Autodesk Inventor part; units mm, degrees
ref_plane "YZ Plane" through (0, 0, 0) normal (1, 0, 0) x (0, 1, 0)
ref_plane "XZ Plane" through (0, 0, 0) normal (0, 1, 0) x (-1, 0, 0)
ref_plane "XY Plane" through (0, 0, 0) normal (0, 0, 1) x (1, 0, 0)
sketch "스케치1" plane through (0, 0, 0) normal (0, 1, 0) x (-1, 0, 0)
  line L0 (-150, 125) -> (-150, -175)
  line L1 (-150, -175) -> (150, -175)
  line L2 (150, -175) -> (150, 125)
  line L3 (150, 125) -> (100, 125)
  line L4 (100, 125) -> (100, 175)
  line L5 (100, 175) -> (-100, 175)
  line L6 (-100, 175) -> (-100, 125)
  line L7 (-100, 125) -> (-150, 125)
  point P0 (0, 0)
  dimension "d3" = 300
  dimension "d4" = 150
  dimension "d8" = 350
  dimension "d10" = 175
  dimension "d11" = 50
extrude "돌출1" add sketch "스케치1" along normal blind 10
sketch "스케치3" plane through (0, 0, 0) normal (0, 0, 1) x (1, 0, 0)
  line L0 (150, 10) -> (-150, 10)
  line L1 (-125, 10) -> (-84.6452, 58.0929)
  line L2 (-59.1104, 70) -> (59.1104, 70)
  line L3 (100, 0) -> (100, 10)
  line L4 (84.6452, 58.0929) -> (125, 10)
  line L5 (0, 0) -> (0, 70)
  arc A0 (-59.1104, 70) -> (-84.6452, 58.0929) centre (-59.1104, 36.6667) ccw
  arc A1 (84.6452, 58.0929) -> (59.1104, 70) centre (59.1104, 36.6667) ccw
  line L6 (125, 10) -> (-125, 10)
  point P0 (-74.654, 70)
  point P1 (74.654, 70)
  point P2 (125, 10)
  dimension "d15" = 130
  dimension "d17" = 33.3333
  dimension "d18" = 33.3333
  dimension "d19" = 300
  dimension "d22" = 250
  dimension "d24" = 60
  dimension "d25" = 0
sketch "스케치4" plane through (0, 0, 0) normal (1, 0, 0) x (0, 1, 0)
  line L0 (70, -175) -> (70, 59.1104)
  line L1 (58.0929, 84.6452) -> (10, 125)
  line L2 (10, 175) -> (10, 125)
  line L3 (10, -175) -> (10, 125)
  line L4 (70, -175) -> (10, -175)
  arc A0 (70, 59.1104) -> (58.0929, 84.6452) centre (36.6667, 59.1104) ccw
  point P0 (0, 0)
  dimension "d27" = 130
  dimension "d28" = 33.3333
  dimension "d29" = 60
extrude "돌출3" add sketch "스케치3" against normal up to surface (175 mm away)
sketch "스케치5" plane through (0, 10, 0) normal (0, 1, 0) x (1, 0, 0)
  line L0 (125, 175) -> (125, 0)
  line L1 (125, 0) -> (-125, 0)
  line L2 (-125, 0) -> (-125, 175)
  line L3 (-125, 175) -> (-150, 175)
  line L4 (-150, 175) -> (-150, -125)
  line L5 (-150, -125) -> (-100, -125)
  line L6 (-100, -125) -> (-100, -175)
  line L7 (-100, -175) -> (100, -175)
  line L8 (100, -175) -> (100, -125)
  line L9 (100, -125) -> (150, -125)
  line L10 (150, -125) -> (150, 175)
  line L11 (150, 175) -> (125, 175)
  line L12 (66, -151) -> (-66, -151)
  line L13 (-76, -141) -> (-76, -111)
  line L14 (-86, -101) -> (-116, -101)
  line L15 (-126, -91) -> (-126, -24)
  line L16 (-126, -24) -> (126, -24)
  line L17 (126, -24) -> (126, -91)
  line L18 (116, -101) -> (86, -101)
  line L19 (76, -111) -> (76, -141)
  arc A0 (86, -101) -> (76, -111) centre (86, -111) ccw
  arc A1 (-76, -111) -> (-86, -101) centre (-86, -111) ccw
  arc A2 (116, -101) -> (126, -91) centre (116, -91) ccw
  arc A3 (-126, -91) -> (-116, -101) centre (-116, -91) ccw
  arc A4 (-76, -141) -> (-66, -151) centre (-66, -141) ccw
  arc A5 (66, -151) -> (76, -141) centre (66, -141) ccw
  point P0 (0, 0)
  dimension "d34" = 24
  dimension "d35" = 10
  dimension "d36" = 10
equation "\"d17\" = 0.5 * d14"
equation "\"d18\" = d17"
equation "\"d22\" = 0.833333 * d19"
equation "\"d24\" = 0.2 * d19"
equation "\"d27\" = d15"
equation "\"d28\" = d17"
equation "\"d29\" = d24"
equation "\"d36\" = d35"
equation "\"d14\" = 0.333333 * d16"
properties part number "cap2"
Design review of the part built by this model. Coordinates are the model's own, in mm. A direction names the side the tool comes from. Give positions to 0.01 mm unless a question says otherwise; leave off trailing zeros. Order: outer loops, then holes, each group sorted by start corner. A loop starts at its lowest first (then second) coordinate and runs counter-clockwise, first axis right, second up. Notation, with made-up numbers: (72, 24) -> (89, 24) arc R14 cw to (89, 48) -> close; hole circle Ø7 at (36, 14.25). An arc over 180 degrees is marked (long way). Write each question's results on one line, items separated by ' | '. Start each with the question number.
Q1. Add section A-A on z = -97.5. Give the boundary of the cut face in (x, y), and give its area (3 significant figures).
Q2. Machinability: for faces 1 (the flat face through (125, 5, 125)), 2 (the flat face through (-2, 40, 0)), 3 (the flat face through (-100, 5, 150)), which of the approach directions +Z, -Z, +X, -X, +Y, -Y give a long, thin tool a straight path to every point of the face, cutting with its end or side? Answer none if there is none.
Q3. Add section D-D on z = 145.5. Give the boundary of the cut face in (x, y).
Q4. Add section C-C on y = 19. Give the boundary of the cut face in (x, z).
Q5. For pin 1 (3 mm diameter, centred on x = 14.5, z = 24.5, fed in from +Y); pin 2 (11 mm diameter, centred on y = 5, z = 142.5, fed in from -X); pin 3 (11 mm diameter, centred on x = 119, y = 6.5, fed in from +Z), all flat-tipped, find the tip position at first contact; note any pin that passes through.
Q6. Add section B-B on x = 14.5. Give the boundary of the cut face in (y, z).
Q7. Wall thickness on L1, parallel to Z at x = -46, y = 65; L2, parallel to Y at x = -61, z = -128.5; L3, parallel to Y at x = -49.5, z = 100: over which ranges is each line inside the solid? List them lowest first. Write a range as from..to.
Found:
1) outline: (-150, 0) -> (150, 0) -> (150, 10) -> (125, 10) -> (84.65, 58.09) arc R33.33 ccw to (59.11, 70) -> (-59.11, 70) arc R33.33 ccw to (-84.65, 58.09) -> (-125, 10) -> (-150, 10) -> close | area: 14,900 mm2
2) face 1: +Z, +X, +Y, -Y | face 2: +Z, +X, -X, +Y | face 3: +Z, -X, +Y, -Y
3) outline: (-100, 0) -> (100, 0) -> (100, 10) -> (-100, 10) -> close
4) outline: (-117.45, -175) -> (117.45, -175) -> (117.45, 0) -> (-117.45, 0) -> close
5) pin 1: stops at y = 10 | pin 2: stops at x = -100 | pin 3: stops at z = 125
6) outline: (0, -175) -> (70, -175) -> (70, 0) -> (10, 0) -> (10, 175) -> (0, 175) -> close
7) L1: z = -175..0 | L2: y = 0..69.95 | L3: y = 0..10
